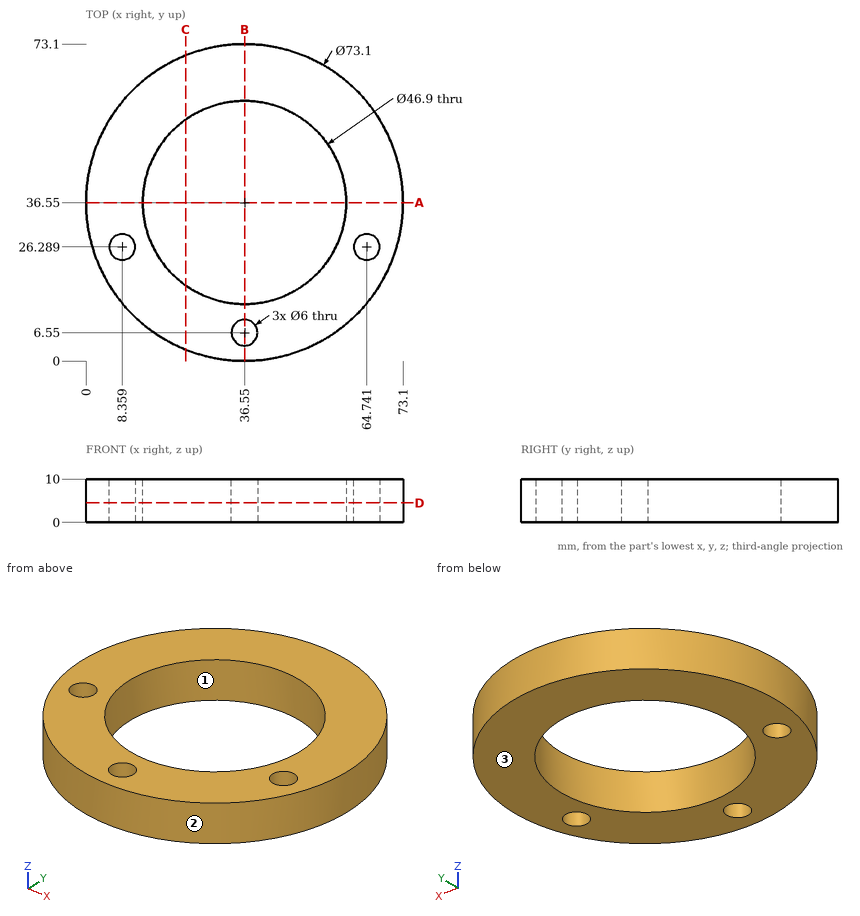
Source: three-view drawing plus pictorial views. Frame: mm from the lowest corner of the part. Round coordinates to 2 decimals unless told otherwise and drop trailing zeros. Loops run counter-clockwise (first coordinate to the right, second up) from the corner with the lowest first, then second, coordinate; pieces in that order, holes last.
Q1. Section D-D, the plane z = 4.5. Return loops of the section in (x, y), plus the area to 3 significant figures.
Q2. Ray query, line 1 (Y direction, x = 36.55, z = 7); line 2 (X direction, y = 36.55, z = 2.75); line 3 (X direction, y = 34, z = 8). Return the intervals inside material, ascending.
Q3. Section A-A, the plane y = 36.55. Return loops of the section in (x, z).
Q4. First-contact query: P1, Ø3, axis at x = 14.5, z = 3, coming from the -Y side (1 decimal); P2, Ø1, axis at x = 18.5, z = 6.5, coming from the -Y side; P3, Ø5, axis at y = 52, z = 2, coming from the +X side. Flat tips, straight axial feed; report the tip coordinate or a pass-through.
Q5. Section B-B, the plane x = 36.55. Return loops of the section in (y, z), plus the area to 3 significant figures.
Q6. Mould query, pull axis Y, two halves, no side actions, for the marked faces 1, 2 and 3. Classes: pulls with the +Y half, pulls with the -Y half, needs draft (parallel to the pull), parting line crosses it, or undercut.
Q7. Section C-C, the plane x = 23. Return loops of the section in (y, z) (1 decimal).
Solutions:
1. outline: circle Ø73.1 at (36.55, 36.55); hole circle Ø6 at (8.36, 26.29); hole circle Ø46.9 at (36.55, 36.55); hole circle Ø6 at (36.55, 6.55); hole circle Ø6 at (64.74, 26.29)
1. area: 2,380 mm2
2. line 1: y = 0 to 3.55, 9.55 to 13.1, 60 to 73.1
2. line 2: x = 0 to 13.1, 60 to 73.1
2. line 3: x = 0.09 to 13.24, 59.86 to 73.01
3. outline: (0, 0) - (13.1, 0) - (13.1, 10) - (0, 10) - close; (60, 0) - (73.1, 0) - (73.1, 10) - (60, 10) - close
4. P1: stops at y = 6.3
4. P2: stops at y = 4.49
4. P3: stops at x = 70.73
5. outline: (0, 0) - (3.55, 0) - (3.55, 10) - (0, 10) - close; (9.55, 0) - (13.1, 0) - (13.1, 10) - (9.55, 10) - close; (60, 0) - (73.1, 0) - (73.1, 10) - (60, 10) - close
5. area: 202 mm2
6. face 1: undercut
6. face 2: parting line crosses it
6. face 3: needs draft
7. outline: (2.6, 0) - (17.4, 0) - (17.4, 10) - (2.6, 10) - close; (55.7, 0) - (70.5, 0) - (70.5, 10) - (55.7, 10) - close
